from build123d import *

# Parameters (mm, degrees)
SKETCH1_W            = 200
SKETCH1_H            = 80
BOSS_EXTRUDE1_DEPTH  = 30
CHAMFER1_SIZE        = 10
SKETCH2_R            = 1
CUT_EXTRUDE1_DEPTH   = 40
LPATTERN1_COUNT      = 3
LPATTERN1_PITCH      = 152
LPATTERN1_COUNT_DIR2 = 2
LPATTERN1_PITCH_DIR2 = 31


with BuildPart() as part:
    # Sketch1 → Boss-Extrude1 (new body)
    with BuildSketch(Plane(origin=(0, 0, 0), x_dir=(1, 0, 0), z_dir=(0, 1, 0))):
        with Locations((-74.550128535, 27.789203085)):
            Rectangle(SKETCH1_W, SKETCH1_H)
    extrude(amount=BOSS_EXTRUDE1_DEPTH)

    # Chamfer1
    chamfer1_edges = [part.edges().sort_by_distance(p)[0] for p in [
        (-174.550128535, 30, -27.789203085),
        (-74.550128535, 30, 12.210796915),
        (25.449871465, 30, -27.789203085),
        (-74.550128535, 30, -67.789203085),
    ]]
    chamfer(chamfer1_edges, length=CHAMFER1_SIZE)

    # Sketch2 → Cut-Extrude1 (cut)
    with BuildSketch(Plane(origin=(0, 30, 0), x_dir=(1, 0, 0), z_dir=(0, 1, 0))):
        with Locations(Location((1.449871465, 43.289203085, 0), (0, 0, 270))):
            Circle(SKETCH2_R)
    cut_extrude1 = extrude(amount=-CUT_EXTRUDE1_DEPTH, mode=Mode.SUBTRACT)

    # LPattern1: Cut-Extrude1 3 × 2
    with Locations(*[(-i * LPATTERN1_PITCH, 0, j * LPATTERN1_PITCH_DIR2) for i in range(LPATTERN1_COUNT) for j in range(LPATTERN1_COUNT_DIR2) if (i, j) != (0, 0)]):
        add(cut_extrude1, mode=Mode.SUBTRACT)


solid = part.part
Build history of the part. All positions in model axes, mm. Give positions to 0.01 mm unless a question says otherwise; leave off trailing zeros. Write each loop counter-clockwise with the first axis right and the second up, starting at its lowest first coordinate (ties: lowest second). Pieces come first, ordered by that corner, then holes. Notation, with made-up numbers: (-24, 2) - (27, 2) arc R21 cw to (27, 7) - close; hole circle Ø10 at (-36, 67.5). An arc over 180 degrees is marked (long way). Use one line per item in the form item = value. Start each with the question number.
1. Drop flat-ended pins along their axis: pin 1 Ø1.6 at (x, z) = (-150.55, -43.29) entering from +Y; pin 2 Ø8 at (x, y) = (-86.5, 27) entering from -Z; pin 3 Ø1 at (y, z) = (27, 4) entering from +X. Give the stop position or say it passes through.
2. Band-saw the part on A-A on z = -19.5. Write the cut outline in (x, y), plus the area to 3 significant figures.
3. Probe line 1 (Z direction, x = -24, y = 23); line 2 (X direction, y = 25.25, z = -31.5); line 3 (X direction, y = 25.75, z = 0). List the from-to ranges inside material, lowest first. Write a range as [from, to].
4. Band-saw the part on C-C on x = -118.5. Write the cut outline in (y, z).
5. Band-saw the part on B-B on y = 27. Write the cut outline in (x, z).
Conclusion:
q1.pin_1 = through
q1.pin_2 = -64.79
q1.pin_3 = 18.95
q2.outline = (-174.55, 0) - (25.45, 0) - (25.45, 20) - (15.45, 30) - (-164.55, 30) - (-174.55, 20) - close
q2.area = 5,900 mm²
q3.line_1 = [-64.79, 9.21]
q3.line_2 = [-169.3, 20.2]
q3.line_3 = [-168.8, 19.7]
q4.outline = (0, -67.79) - (20, -67.79) - (30, -57.79) - (30, 2.21) - (20, 12.21) - (0, 12.21) - close
q5.outline = (-167.55, -60.79) - (18.45, -60.79) - (18.45, 5.21) - (-167.55, 5.21) - close; hole circle Ø2 at (-150.55, -43.29); hole circle Ø2 at (-150.55, -12.29); hole circle Ø2 at (1.45, -43.29); hole circle Ø2 at (1.45, -12.29)
